```python
from build123d import *

# Parameters (mm, degrees)
ESQUISSE1_R        = 1.6
BOSS_EXTRU_1_DEPTH = 3


with BuildPart() as part:
    # Esquisse1 → Boss.-Extru.1 (new body)
    with BuildSketch(Plane.XY):
        Polygon((-106.057456456, -118.225792128), (-128.094157446, -96.85509979), (-131.150893181, -96.85509979), (-131.679198628, -95.012679745), (-203.911321115, -95.012679745), (-204.439626562, -96.85509979), (-207.491865187, -96.85509979), (-208.236606037, -97.572971364), (-229.533063287, -118.225792128), (-242.655085998, -104.673746846), (-258.969310369, -95.012679745), (-277.629290011, -88.825419148), (-272.289144354, -70.202118055), (-298.538981418, -62.6750984), (-299.849714513, -67.246167925), (-337.461409717, -56.461187875), (-321.404434006, -0.463858857), (-284.873898651, -10.938821309), (-283.564528345, -6.372504389), (-265.299260667, -11.609985616), (-264.679553884, -9.448811229), (-245.452786066, -14.960840928), (-246.072799476, -17.123084647), (-227.807531798, -22.360565873), (-228.496674065, -24.763890567), (-209.275142378, -30.275576085), (-204.23586614, -12.701531345), (-206.165691337, -12.701531345), (-221.686141291, -8.251113935), (-228.411595336, -6.322621021), (-237.526398495, -3.709541892), (-245.374022141, -1.459744369), (-249.872259625, -3.248768002), (-288.323340616, 7.774587685), (-291.190458161, 11.675149567), (-324.146226634, 21.123080509), (-329.606279511, 18.096325283), (-352.324375235, -61.131089881), (-349.297882974, -66.591026451), (-293.334748244, -82.638197107), (-287.498708924, -98.561018129), (-250.280154874, -115.48724507), (-232.892593163, -133.444615579), (-226.653475651, -133.542771169), (-198.570548361, -106.350948678), (-137.019971382, -106.350948678), (-108.937044092, -133.542771169), (-102.69792658, -133.444615579), (-85.310364869, -115.48724507), (-48.091810819, -98.561018129), (-42.255771499, -82.638197107), (13.707363231, -66.591026451), (16.733855492, -61.131089881), (-5.984240232, 18.096325283), (-11.444293109, 21.123080509), (-44.400061582, 11.675149567), (-47.267179127, 7.774587685), (-85.718260118, -3.248768002), (-90.216497602, -1.459744369), (-98.064121248, -3.709541892), (-107.178924407, -6.322621021), (-113.904378452, -8.251113935), (-129.424828406, -12.701531345), (-180.308979115, -12.701531345), (-196.245732321, -68.279594663), (-194.797007033, -70.202118055), (-140.79351271, -70.202118055), (-139.344787422, -68.279594663), (-147.87312166, -38.537758661), (-146.501872979, -36.063960558), (-107.093845678, -24.763890567), (-107.782987945, -22.360565873), (-89.517720268, -17.123084647), (-90.137733677, -14.960840928), (-70.910965859, -9.448811229), (-70.291259076, -11.609985616), (-52.025991399, -6.372504389), (-50.716621092, -10.938821309), (-14.186085737, -0.463858857), (1.870889973, -56.461187875), (-35.740805231, -67.246167925), (-37.051538325, -62.6750984), (-63.301375389, -70.202118055), (-57.961229733, -88.825419148), (-76.621209374, -95.012679745), (-92.935433745, -104.673746846), align=None)
        with Locations((-229.666591606, -126.713325795)):
            Circle(ESQUISSE1_R, mode=Mode.SUBTRACT)
        with Locations((-204.059552706, -101.880200807)):
            Circle(ESQUISSE1_R, mode=Mode.SUBTRACT)
        with Locations((-281.934339477, -93.401689518)):
            Circle(ESQUISSE1_R, mode=Mode.SUBTRACT)
        with Locations((-344.882804027, -60.574933915)):
            Circle(ESQUISSE1_R, mode=Mode.SUBTRACT)
        with Locations((-105.923928137, -126.713325795)):
            Circle(ESQUISSE1_R, mode=Mode.SUBTRACT)
        with Locations((-131.530967037, -101.880200807)):
            Circle(ESQUISSE1_R, mode=Mode.SUBTRACT)
        with Locations((-53.656180266, -93.401689518)):
            Circle(ESQUISSE1_R, mode=Mode.SUBTRACT)
        with Locations((9.292284284, -60.574933915)):
            Circle(ESQUISSE1_R, mode=Mode.SUBTRACT)
        with Locations((-167.795259872, -27.605548894)):
            Circle(ESQUISSE1_R, mode=Mode.SUBTRACT)
        with Locations((-323.590068827, 13.68165837)):
            Circle(ESQUISSE1_R, mode=Mode.SUBTRACT)
        with Locations((-216.832585966, -16.924131519)):
            Circle(ESQUISSE1_R, mode=Mode.SUBTRACT)
        with Locations((-118.757933777, -16.924131519)):
            Circle(ESQUISSE1_R, mode=Mode.SUBTRACT)
        with Locations((-12.000450916, 13.68165837)):
            Circle(ESQUISSE1_R, mode=Mode.SUBTRACT)
    extrude(amount=BOSS_EXTRU_1_DEPTH)


solid = part.part
```
Can you work these out from the model? Positions are in its coordinate system, mm. A direction names the side the tool comes from. Give positions to 0.01 mm unless a question says otherwise; leave off trailing zeros. Write each loop counter-clockwise with the first axis right and the second up, starting at its lowest first coordinate (ties: lowest second). Pieces come first, ordered by that corner, then holes. Notation, with made-up numbers: (-1, 64.5) - (42, 64.5) arc R26 cw to (42, 83.5) - close; hole circle Ø8 at (1.25, 0.5). An arc over 180 degrees is marked (long way). Write item = value, one per line. Start each with the question number.
1. On a 3-axis mill with a long thin cutter (end or side, diameter ignored), from which of +Z, -Z, +X, -X, +Y, -Y can I reach the whole of each face in a straight line? I mean faces 5 (the face through (-67.161, -91.876, 1.479)), 6 (the face through (-307.438, 16.333, 1.479)), 7 (the face through (-123.175, -119.757, 1.479)). Say none if no direction works.
2. Imagine slicing it at C-C (z = 2.25). Count the separate pieces of the cut face and the enclosed holes in it, and give its area (3 significant figures).
3. For pin 1 (4 mm diameter, centred on x = 9.29, y = -60.57, fed in from -Z); pin 2 (1.5 mm diameter, centred on y = -41.5, z = 2, fed in from -X); pin 3 (1.5 mm diameter, centred on x = -164.5, z = 2, fed in from -Y); pin 4 (1.5 mm diameter, centred on x = -205, z = 2, fed in from +Y), each with a flat end and sliding along its axis, tell me the tip position at first contact or that it passes through.
4. Please list where these lines run through material, in increasing order: line 1 (X direction, y = -103, z = 1.6); line 2 (Y direction, x = -173, z = 2.7); line 3 (Y direction, x = -132, z = 1.75).
5. Imagine slicing it at B-B (y = -50.5). Please give me the cut outline in (x, z).
6. Thinking about a two-plate mould opening in Y: for faces 1 (the face through (-14.67, -74.73, 1.48)), 2 (the face through (-49.993, -66.386, 1.479)), 3 (the face through (-169, -50, 3)), 4 (the face through (-99.4, -111.35, 1.48)), which applies, released by +Y, released by -Y, zero draft, split by the parting line, or undercut?
7. Imagine slicing it at A-A (x = -173). Please give me the cut outline in (y, z), and give its area (3 significant figures).
Worked answers:
q1.face_5 = +Z, -Z
q1.face_6 = +Z, -Z, +Y
q1.face_7 = +Z, -Z, -Y
q2.separate_pieces = 1
q2.enclosed_holes = 13
q2.area = 14,500 mm2
q3.pin_1 = 0
q3.pin_2 = -346.91
q3.pin_3 = -106.35
q3.pin_4 = -12.7
q4.line_1 = -277.74 to -245.48, -213.83 to -205.2, -202.92 to -132.67, -130.39 to -121.76, -90.11 to -57.85
q4.line_2 = -106.35 to -95.01, -70.2 to -12.7
q4.line_3 = -111.21 to -103.41, -100.35 to -95.01, -31.91 to -12.7
q5.outline = (-349.28, 0) - (-335.75, 0) - (-335.75, 3) - (-349.28, 3) - close; (-191.15, 0) - (-144.44, 0) - (-144.44, 3) - (-191.15, 3) - close; (0.16, 0) - (13.69, 0) - (13.69, 3) - (0.16, 3) - close
q6.face_1 = released by -Y
q6.face_2 = undercut
q6.face_3 = zero draft
q6.face_4 = undercut
q7.outline = (-106.35, 0) - (-95.01, 0) - (-95.01, 3) - (-106.35, 3) - close; (-70.2, 0) - (-12.7, 0) - (-12.7, 3) - (-70.2, 3) - close
q7.area = 207 mm2
